```python
from build123d import *

# Parameters (mm, degrees)
SKETCH_W     = 9
SKETCH_H     = 11
PAD_DEPTH    = 3.5
PAD001_DEPTH = 13.5
SKETCH002_R  = 3
POCKET_DEPTH = 11
FILLET_R     = 0.1


with BuildPart() as part:
    # Sketch → Pad (new body)
    with BuildSketch(Plane.XZ):
        with Locations((0, -1)):
            Rectangle(SKETCH_W, SKETCH_H)
    extrude(amount=-PAD_DEPTH)

    # Sketch001 (on Face5 of Pad) → Pad001 (join)
    with BuildSketch(Plane.XZ):
        with BuildLine():
            Line((-4.5, -6.5), (4.5, -6.5))
            Line((4.5, -6.5), (4.5, 0))
            Line((4.5, 0), (4.3, 0))
            ThreePointArc((4.3, 0), (0, 4.3), (-4.3, 0))
            Line((-4.5, 0), (-4.3, 0))
            Line((-4.5, 0), (-4.5, -6.5))
        make_face()
    extrude(amount=-PAD001_DEPTH)

    # Sketch002 (on Face8 of Pad001) → Pocket (cut)
    with BuildSketch(Plane.XZ):
        Circle(SKETCH002_R)
    extrude(amount=-POCKET_DEPTH, mode=Mode.SUBTRACT)

    # Fillet
    fillet_edges = [part.edges().sort_by_distance(p)[0] for p in [
        (0, 0, 4.5),
        (4.5, 1.75, 4.5),
        (0, 3.5, 4.5),
        (-4.5, 1.75, 4.5),
        (4.5, 0, 2.25),
        (-4.5, 0, 2.25),
        (0, 0, -6.5),
        (-3, 0, 0),
    ]]
    fillet(fillet_edges, radius=FILLET_R)


solid = part.part
```
Work out the finished part from the listing and answer in its coordinate system (mm). A direction names the side the tool comes from. Give positions to 0.01 mm unless a question says otherwise; leave off trailing zeros. Order: outer loops, then holes, each group sorted by start corner. A loop starts at its lowest first (then second) coordinate and runs counter-clockwise, first axis right, second up. Notation, with made-up numbers: (53, -7) -> (75, -7) arc R33 ccw to (75, 32) -> close; hole circle Ø1 at (68, -18.5). An arc over 180 degrees is marked (long way). Answer as CSV lines item,"result". Start each with the question number.
(1) For a pull along X with two mould halves and no side action, classify faces 1 (the flat face through (-4.5, 5, -2)), 2 (the cylindrical face through (-3, 5, 0)), 3 (the flat face through (0, 13.5, -1)), 4 (the flat face through (4.5, 5, -2)) as released by +X, released by -X, zero draft, split by the parting line, or undercut.
(2) Each of these flat-tipped pins is pushed along its axis until it touches: pin 1 Ø5 at (x, z) = (0, 0) entering from -Y; pin 2 Ø2 at (x, y) = (-1, 9.5) entering from +Z. Where does it stop, or does it pass through?
(3) Section A-A, the plane y = 9 is taken. Write down the section's boundary in (x, z), plus the area to 3 significant figures.
(4) Consider line 1 along Z through (x, y) = (0, 8); line 2 along Y through (x, z) = (1, 2); line 3 along X through (y, z) = (10.5, -2). Determine where each line is inside the solid, lowest interval first.
(5) Which of the six approach directions +Z, -Z, +X, -X, +Y, -Y give full straight-line access (tool end or side, diameter ignored) to faces 5 (the flat face through (0, 11, 0)), 6 (the flat face through (-2, 3.5, 4)), 7 (the flat face through (0, 2, 4.5))?
(6) Section B-B, the plane x = 0 is taken. Write down the section's boundary in (y, z).
Entries:
1,face 1,"released by -X"
1,face 2,"undercut"
1,face 3,"zero draft"
1,face 4,"released by +X"
2,pin 1,"y = 11"
2,pin 2,"z = 4.3"
3,outline,"(-4.5, -6.5) -> (4.5, -6.5) -> (4.5, 0) -> (4.3, 0) arc R4.3 ccw to (-4.3, 0) -> (-4.5, 0) -> close; hole circle Ø6 at (0, 0)"
3,area,"59.3 mm²"
4,line 1,"-6.5 to -3, 3 to 4.3"
4,line 2,"11 to 13.5"
4,line 3,"-4.5 to -2.24, 2.24 to 4.5"
5,face 5,"-Y"
5,face 6,"+Z, +Y"
5,face 7,"+Z, +X, -X, +Y, -Y"
6,outline,"(0, -6.4) arc R0.1 ccw to (0.1, -6.5) -> (13.5, -6.5) -> (13.5, 4.3) -> (3.5, 4.3) -> (3.5, 4.4) arc R0.1 ccw to (3.4, 4.5) -> (0.1, 4.5) arc R0.1 ccw to (0, 4.4) -> (0, 3.1) arc R0.1 ccw to (0.1, 3) -> (11, 3) -> (11, -3) -> (0.1, -3) arc R0.1 ccw to (0, -3.1) -> close"
